Autodesk Inventor part; units mm, degrees
ref_plane "YZ Plane" through (0, 0, 0) normal (1, 0, 0) x (0, 1, 0)
ref_plane "XZ Plane" through (0, 0, 0) normal (0, 1, 0) x (-1, 0, 0)
ref_plane "XY Plane" through (0, 0, 0) normal (0, 0, 1) x (1, 0, 0)
sketch "Sketch1" plane through (0, 0, 0) normal (0, 1, 0) x (-1, 0, 0)
  line L0 (8.89, 0) -> (-8.89, 0) construction
  line L1 (8.89, 1.5875) -> (-8.89, 1.5875)
  line L2 (-8.89, -1.5875) -> (8.89, -1.5875)
  arc A0 (8.89, -1.5875) -> (8.89, 1.5875) centre (8.89, 0) ccw
  arc A1 (-8.89, 1.5875) -> (-8.89, -1.5875) centre (-8.89, 0) ccw
  line L3 (8.89, -5.0038) -> (-8.89, -5.0038) construction
  line L4 (8.89, -3.4163) -> (-8.89, -3.4163)
  line L5 (-8.89, -6.5913) -> (8.89, -6.5913)
  arc A2 (8.89, -6.5913) -> (8.89, -3.4163) centre (8.89, -5.0038) ccw
  arc A3 (-8.89, -3.4163) -> (-8.89, -6.5913) centre (-8.89, -5.0038) ccw
  line L6 (8.89, -10.0076) -> (-8.89, -10.0076) construction
  line L7 (8.89, -8.4201) -> (-8.89, -8.4201)
  line L8 (-8.89, -11.5951) -> (8.89, -11.5951)
  arc A4 (8.89, -11.5951) -> (8.89, -8.4201) centre (8.89, -10.0076) ccw
  arc A5 (-8.89, -8.4201) -> (-8.89, -11.5951) centre (-8.89, -10.0076) ccw
  line L9 (12.7, 32.8549) -> (-12.7, 32.8549)
  line L10 (-12.7, 32.8549) -> (-12.7, -17.9451)
  line L11 (-12.7, -17.9451) -> (12.7, -17.9451)
  line L12 (12.7, -17.9451) -> (12.7, 32.8549)
  line L13 (6.35, 26.5049) -> (-6.35, 26.5049) construction
  arc A6 (8.89, -16.5989) -> (8.89, -13.4239) centre (8.89, -15.0114) ccw
  line L14 (-8.89, -16.5989) -> (8.89, -16.5989)
  arc A7 (-8.89, -13.4239) -> (-8.89, -16.5989) centre (-8.89, -15.0114) ccw
  line L15 (8.89, -13.4239) -> (-8.89, -13.4239)
  point P0 (0, 0)
  point P1 (0, -5.0038)
  point P2 (0, -10.0076)
  point P3 (10.4775, -5.0038)
  point P4 (10.4775, 0)
  point P5 (10.4775, -10.0076)
  point P6 (0, -17.9451)
  point P7 (0, -11.5951)
  point P8 (0, 26.5049)
  point P9 (0, 32.8549)
  point P10 (10.4775, -15.0114)
  point P11 (0, -16.5989)
  dimension "d1" = 17.78
  dimension "d3" = 3.175
  dimension "d4" = 5.0038
  dimension "d5" = 5.0038
  dimension "d8" = 25.4
  dimension "d9" = 50.8
  dimension "d10" = 6.35
  dimension "d11" = 12.7
  dimension "d12" = 6.35
  dimension "d43" = 5.0038
extrude "Extrusion1" add sketch "Sketch1" along normal blind 3.175 contours A0 L2 A1 L1 | A2 L5 A3 L4 | A4 L8 A5 L7 | L12 L11 L10 L9 | L14 A7 L15 A6
fillet "Fillet1" radius 3.175 4 edges at (-12.7, 1.5875, -17.9451) (12.7, 1.5875, -17.9451) (12.7, 1.5875, 32.8549) (-12.7, 1.5875, 32.8549)
sketch "Sketch2" plane through (0, 3.175, 0) normal (0, 1, 0) x (1, 0, 0)
  line L0 (-6.35, -10.6299) -> (-6.35, -23.3299) construction
  line L1 (-8.9027, -10.6299) -> (-8.9027, -23.3299)
  line L2 (-3.7973, -23.3299) -> (-3.7973, -10.6299)
  arc A0 (-3.7973, -10.6299) -> (-8.9027, -10.6299) centre (-6.35, -10.6299) ccw
  arc A1 (-8.9027, -23.3299) -> (-3.7973, -23.3299) centre (-6.35, -23.3299) ccw
  line L3 (6.35, -10.6299) -> (6.35, -23.3299) construction
  line L4 (3.7973, -10.6299) -> (3.7973, -23.3299)
  line L5 (8.9027, -23.3299) -> (8.9027, -10.6299)
  arc A2 (8.9027, -10.6299) -> (3.7973, -10.6299) centre (6.35, -10.6299) ccw
  arc A3 (3.7973, -23.3299) -> (8.9027, -23.3299) centre (6.35, -23.3299) ccw
  line L6 (-9.525, -32.8549) -> (9.525, -32.8549)
  line L7 (9.525, 17.9451) -> (-9.525, 17.9451)
  line L8 (-6.35, -16.9799) -> (6.35, -16.9799) construction
  point P0 (0, 0)
  point P1 (0, -16.9799)
  point P2 (0, 17.9451)
  dimension "d23" = 5.1054
  dimension "d24" = 12.7
  dimension "d26" = 34.925
  dimension "d27" = 12.7
extrude "Extrusion2" cut sketch "Sketch2" against normal blind 25.4
sketch "Sketch3" plane through (0, 3.175, 0) normal (0, 1, 0) x (1, 0, 0)
  circle A0 centre (0, -45.5549) radius 16.002
  line L0 (-9.525, -32.8549) -> (9.525, -32.8549)
  circle A1 centre (0, -45.5549) radius 19.177
  line L1 (3.7973, -10.6299) -> (3.7973, -23.3299)
  arc A2 (3.7973, -23.3299) -> (8.9027, -23.3299) centre (6.35, -23.3299) ccw
  line L2 (8.9027, -23.3299) -> (8.9027, -10.6299)
  arc A3 (8.9027, -10.6299) -> (3.7973, -10.6299) centre (6.35, -10.6299) ccw
  line L3 (-8.9027, -10.6299) -> (-8.9027, -23.3299)
  arc A4 (-8.9027, -23.3299) -> (-3.7973, -23.3299) centre (-6.35, -23.3299) ccw
  line L4 (-3.7973, -23.3299) -> (-3.7973, -10.6299)
  arc A5 (-3.7973, -10.6299) -> (-8.9027, -10.6299) centre (-6.35, -10.6299) ccw
  arc A6 (-12.7, -29.6799) -> (-9.525, -32.8549) centre (-9.525, -29.6799) ccw
  line L5 (-12.7, -29.6799) -> (-12.7, 14.7701)
  arc A7 (-9.525, 17.9451) -> (-12.7, 14.7701) centre (-9.525, 14.7701) ccw
  line L6 (-9.525, 17.9451) -> (9.525, 17.9451)
  arc A8 (12.7, 14.7701) -> (9.525, 17.9451) centre (9.525, 14.7701) ccw
  line L7 (12.7, 14.7701) -> (12.7, -29.6799)
  arc A9 (9.525, -32.8549) -> (12.7, -29.6799) centre (9.525, -29.6799) ccw
  line L8 (9.525, -32.8549) -> (-9.525, -32.8549)
  line L9 (3.7973, -10.6299) -> (3.7973, -23.3299)
  arc A10 (3.7973, -23.3299) -> (8.9027, -23.3299) centre (6.35, -23.3299) ccw
  line L10 (8.9027, -23.3299) -> (8.9027, -10.6299)
  arc A11 (8.9027, -10.6299) -> (3.7973, -10.6299) centre (6.35, -10.6299) ccw
  line L11 (-8.9027, -10.6299) -> (-8.9027, -23.3299)
  arc A12 (-8.9027, -23.3299) -> (-3.7973, -23.3299) centre (-6.35, -23.3299) ccw
  line L12 (-3.7973, -23.3299) -> (-3.7973, -10.6299)
  arc A13 (-3.7973, -10.6299) -> (-8.9027, -10.6299) centre (-6.35, -10.6299) ccw
  arc A14 (-12.7, -29.6799) -> (-9.525, -32.8549) centre (-9.525, -29.6799) ccw
  line L13 (-12.7, -29.6799) -> (-12.7, 14.7701)
  arc A15 (-9.525, 17.9451) -> (-12.7, 14.7701) centre (-9.525, 14.7701) ccw
  line L14 (-9.525, 17.9451) -> (9.525, 17.9451)
  arc A16 (12.7, 14.7701) -> (9.525, 17.9451) centre (9.525, 14.7701) ccw
  line L15 (12.7, 14.7701) -> (12.7, -29.6799)
  arc A17 (9.525, -32.8549) -> (12.7, -29.6799) centre (9.525, -29.6799) ccw
  line L16 (9.525, -32.8549) -> (-9.525, -32.8549)
  point P0 (0, 0)
  point P1 (0, -32.8549)
  point P2 (12.433, -30.9543)
  point P3 (9.7268, -32.8485)
  point P4 (-9.7268, -32.8485)
  point P5 (-12.433, -30.9543)
  dimension "d30" = 32.004
  dimension "d31" = 12.7
  dimension "d32" = 3.175
sketch "Sketch4" plane through (0, 3.175, 0) normal (0, 1, 0) x (1, 0, 0)
  circle A0 centre (0, -60.4901) radius 1.1811
  arc A1 (-8.5911, -32.8549) -> (-10.7176, -33.6722) centre (-8.5911, -36.0299) ccw
  arc A2 (-10.7176, -33.6722) -> (10.7176, -33.6722) centre (0, -45.5549) ccw
  arc A3 (10.7176, -33.6722) -> (8.5911, -32.8549) centre (8.5911, -36.0299) ccw
  line L0 (8.5911, -32.8549) -> (-8.5911, -32.8549)
  arc A4 (12.6992, -29.749) -> (13.6187, -32.0535) centre (15.8735, -29.8182) ccw
  arc A5 (-13.6187, -32.0535) -> (13.6187, -32.0535) centre (0, -45.5549) ccw
  arc A6 (-13.6187, -32.0535) -> (-12.6992, -29.749) centre (-15.8735, -29.8182) ccw
  arc A7 (-12.7, -29.6799) -> (-12.6992, -29.749) centre (-9.525, -29.6799) ccw
  line L1 (-12.7, -29.6799) -> (-12.7, 14.7701)
  arc A8 (-9.525, 17.9451) -> (-12.7, 14.7701) centre (-9.525, 14.7701) ccw
  line L2 (-9.525, 17.9451) -> (9.525, 17.9451)
  arc A9 (12.7, 14.7701) -> (9.525, 17.9451) centre (9.525, 14.7701) ccw
  line L3 (12.7, 14.7701) -> (12.7, -29.6799)
  arc A10 (12.6992, -29.749) -> (12.7, -29.6799) centre (9.525, -29.6799) ccw
  line L4 (3.7973, -10.6299) -> (3.7973, -23.3299)
  arc A11 (3.7973, -23.3299) -> (8.9027, -23.3299) centre (6.35, -23.3299) ccw
  line L5 (8.9027, -23.3299) -> (8.9027, -10.6299)
  arc A12 (8.9027, -10.6299) -> (3.7973, -10.6299) centre (6.35, -10.6299) ccw
  line L6 (-8.9027, -10.6299) -> (-8.9027, -23.3299)
  arc A13 (-8.9027, -23.3299) -> (-3.7973, -23.3299) centre (-6.35, -23.3299) ccw
  line L7 (-3.7973, -23.3299) -> (-3.7973, -10.6299)
  arc A14 (-3.7973, -10.6299) -> (-8.9027, -10.6299) centre (-6.35, -10.6299) ccw
  point P0 (0, 0)
  point P1 (0, -61.5569)
  point P2 (-0.5246, -61.5483)
  point P3 (0.5246, -61.5483)
  dimension "d36" = 2.3622
  dimension "d37" = 1.0668
sketch "Sketch5" plane through (0, 3.175, 0) normal (0, 1, 0) x (1, 0, 0)
  arc A0 (-8.5911, -32.8549) -> (-10.7176, -33.6722) centre (-8.5911, -36.0299) ccw construction
  arc A1 (-10.7176, -33.6722) -> (-4.3651, -60.95) centre (0, -45.5549) ccw construction
  arc A2 (-4.3651, -60.95) -> (-0.9487, -59.7866) centre (-3.499, -57.8954) ccw construction
  arc A3 (0.9487, -59.7866) -> (-0.9487, -59.7866) centre (0, -60.4901) ccw construction
  arc A4 (0.9487, -59.7866) -> (4.3651, -60.95) centre (3.499, -57.8954) ccw construction
  arc A5 (4.3651, -60.95) -> (10.7176, -33.6722) centre (0, -45.5549) ccw construction
  arc A6 (10.7176, -33.6722) -> (8.5911, -32.8549) centre (8.5911, -36.0299) ccw construction
  line L0 (8.5911, -32.8549) -> (-8.5911, -32.8549) construction
  arc A7 (12.6992, -29.749) -> (13.6187, -32.0535) centre (15.8735, -29.8182) ccw construction
  arc A8 (-13.6187, -32.0535) -> (13.6187, -32.0535) centre (0, -45.5549) ccw construction
  arc A9 (-13.6187, -32.0535) -> (-12.6992, -29.749) centre (-15.8735, -29.8182) ccw construction
  arc A10 (-12.7, -29.6799) -> (-12.6992, -29.749) centre (-9.525, -29.6799) ccw construction
  line L1 (-12.7, -29.6799) -> (-12.7, 14.7701) construction
  arc A11 (-9.525, 17.9451) -> (-12.7, 14.7701) centre (-9.525, 14.7701) ccw construction
  line L2 (-9.525, 17.9451) -> (9.525, 17.9451) construction
  arc A12 (12.7, 14.7701) -> (9.525, 17.9451) centre (9.525, 14.7701) ccw construction
  line L3 (12.7, 14.7701) -> (12.7, -29.6799) construction
  arc A13 (12.6992, -29.749) -> (12.7, -29.6799) centre (9.525, -29.6799) ccw construction
  line L4 (3.7973, -10.6299) -> (3.7973, -23.3299) construction
  arc A14 (3.7973, -23.3299) -> (8.9027, -23.3299) centre (6.35, -23.3299) ccw construction
  line L5 (8.9027, -23.3299) -> (8.9027, -10.6299) construction
  arc A15 (8.9027, -10.6299) -> (3.7973, -10.6299) centre (6.35, -10.6299) ccw construction
  line L6 (-8.9027, -10.6299) -> (-8.9027, -23.3299) construction
  arc A16 (-8.9027, -23.3299) -> (-3.7973, -23.3299) centre (-6.35, -23.3299) ccw construction
  line L7 (-3.7973, -23.3299) -> (-3.7973, -10.6299) construction
  arc A17 (-3.7973, -10.6299) -> (-8.9027, -10.6299) centre (-6.35, -10.6299) ccw construction
  line L8 (-22.86, -21.4249) -> (22.86, -21.4249)
  line L9 (22.86, -21.4249) -> (22.86, -69.6849)
  line L10 (22.86, -69.6849) -> (-22.86, -69.6849)
  line L11 (-22.86, -69.6849) -> (-22.86, -21.4249)
  line L12 (-22.86, -21.4249) -> (22.86, -69.6849) construction
  line L13 (22.86, -21.4249) -> (-22.86, -69.6849) construction
  line L14 (-22.86, -41.1099) -> (-12.7, -23.3299)
  line L15 (-12.7, 14.7701) -> (-12.7, -29.6799) construction
  line L16 (12.7, -29.6799) -> (12.7, 14.7701) construction
  line L17 (12.7, -23.3299) -> (22.86, -41.1099)
  arc A18 (-13.6187, -32.0535) -> (-12.6992, -29.749) centre (-15.8735, -29.8182) ccw construction
  arc A19 (-13.6187, -32.0535) -> (13.6187, -32.0535) centre (0, -45.5549) ccw construction
  arc A20 (-13.6187, -32.0535) -> (13.6187, -32.0535) centre (0, -45.5549) ccw
  arc A21 (12.6992, -29.749) -> (13.6187, -32.0535) centre (15.8735, -29.8182) ccw
  arc A22 (-13.5868, -32.0214) -> (-12.6998, -29.7145) centre (-15.8735, -29.8182) ccw
  arc A23 (-12.7, -29.6799) -> (-12.6992, -29.749) centre (-9.525, -29.6799) ccw construction
  line L18 (-13.5868, -32.0214) -> (-13.6187, -32.0535)
  line L19 (-12.7, -23.3299) -> (-12.6998, -29.7145)
  line L20 (12.7, -23.3299) -> (12.7, -29.6799)
  arc A24 (12.6992, -29.749) -> (12.7, -29.6799) centre (9.525, -29.6799) ccw construction
  line L21 (12.7, -29.916) -> (12.7, -29.6799)
  point P0 (0, 0)
  dimension "d48" = 45.72
  dimension "d49" = 87.63
  dimension "d50" = 28.575
equation "\"d43\" = d5"
properties part number "EL2-034" material "Aluminum 6061"
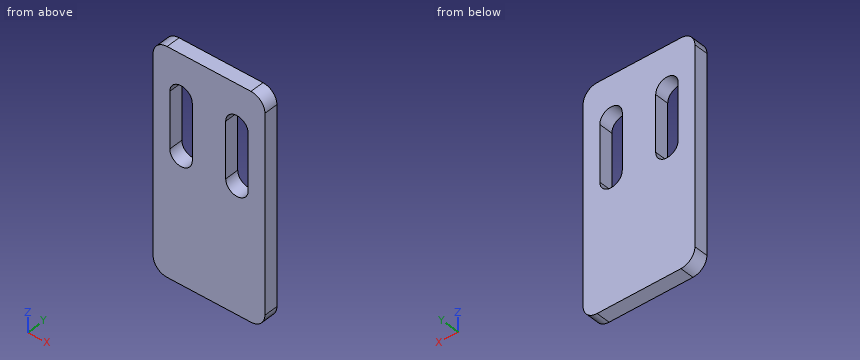
Here's how the part is built. I have some questions about the finished solid (model axes, mm). Give positions to 0.01 mm unless a question says otherwise; leave off trailing zeros. Order: outer loops, then holes, each group sorted by start corner. A loop starts at its lowest first (then second) coordinate and runs counter-clockwise, first axis right, second up. Notation, with made-up numbers: M 70,16 L 120,16 A21 ccw 120,34 Z; hole C -10.75,81.25 d11. An arc over 180 degrees is marked long. Use a Markdown table: item, result. Add a question column.
1. I need wall thicknesses on probe 1 along X at (y, z) = (0.7, 16); probe 2 along X at (y, z) = (0.25, 10); probe 3 along Z at (x, y) = (-6.5, 2.5). Which ranges of each line are inside material? Lowest first, please. Write a range as from..to.
2. Suppose I cut it at D-D (x = -7). List the corners of the cut face in (y, z) for me (3 decimals).
3. Suppose I cut it at A-A (z = 11.5). List the corners of the cut face in (x, y) for me (3 decimals), and give its area (3 significant figures).
4. Suppose I cut it at B-B (y = 1.8). List the corners of the cut face in (x, z) for me (3 decimals).
5. Suppose I cut it at C-C (x = 6.35). List the corners of the cut face in (y, z) for me (3 decimals).
Results list:
| question | item | result |
|---|---|---|
| 1 | probe 1 | x = -12.7..-8.9, -3.8..3.8, 8.9..12.7 |
| 1 | probe 2 | x = -12.7..-8.82, -3.88..3.88, 8.82..12.7 |
| 1 | probe 3 | z = -17.95..8.08, 25.88..32.85 |
| 2 | outline | M 0,-17.945 L 3.175,-17.945 L 3.175,8.161 L 0,8.161 Z; M 0,25.798 L 3.175,25.798 L 3.175,32.855 L 0,32.855 Z |
| 3 | outline | M -12.7,0 L -8.903,0 L -8.903,3.175 L -12.7,3.175 Z; M -3.797,0 L 3.797,0 L 3.797,3.175 L -3.797,3.175 Z; M 8.903,0 L 12.7,0 L 12.7,3.175 L 8.903,3.175 Z |
| 3 | area | 48.2 mm² |
| 4 | outline | M -12.7,-14.77 A3.175 ccw -9.525,-17.945 L 9.525,-17.945 A3.175 ccw 12.7,-14.77 L 12.7,29.68 A3.175 ccw 9.525,32.855 L -9.525,32.855 A3.175 ccw -12.7,29.68 Z; hole M -8.903,10.63 A2.553 ccw -3.797,10.63 L -3.797,23.33 A2.553 ccw -8.903,23.33 Z; hole M 3.797,10.63 A2.553 ccw 8.903,10.63 L 8.903,23.33 A2.553 ccw 3.797,23.33 Z |
| 5 | outline | M 0,-17.945 L 3.175,-17.945 L 3.175,8.077 L 0,8.077 Z; M 0,25.883 L 3.175,25.883 L 3.175,32.855 L 0,32.855 Z |
